from build123d import *

# Parameters (mm, degrees)
SKETCH1_R           = 12.5
SKETCH1_R_2         = 6
SKETCH1_R_3         = 1.5
SKETCH1_R_4         = 3
BOSS_EXTRUDE1_DEPTH = 4.5
BOSS_EXTRUDE2_START = 4.5
SKETCH1_3_R         = 6
SKETCH1_3_R_2       = 3
BOSS_EXTRUDE2_DEPTH = 4.5


with BuildPart() as part:
    # Sketch1 → Boss-Extrude1 (new body)
    # profile 1 of 2: a face of its own
    with BuildSketch(Plane(origin=(0, 0, 0), x_dir=(1, 0, 0), z_dir=(0, 1, 0))):
        with Locations(Location((0, 0, 0), (0, 0, 270))):
            Circle(SKETCH1_R)
        Circle(SKETCH1_R_2, mode=Mode.SUBTRACT)
        with Locations(Location((-8.227241336, 4.75, 0), (0, 0, 270))):
            Circle(SKETCH1_R_3, mode=Mode.SUBTRACT)
        with Locations(Location((-8.227241336, -4.75, 0), (0, 0, 270))):
            Circle(SKETCH1_R_3, mode=Mode.SUBTRACT)
        with Locations(Location((0, -9.5, 0), (0, 0, 270))):
            Circle(SKETCH1_R_3, mode=Mode.SUBTRACT)
        with Locations(Location((8.227241336, -4.75, 0), (0, 0, 270))):
            Circle(SKETCH1_R_3, mode=Mode.SUBTRACT)
        with Locations(Location((8.227241336, 4.75, 0), (0, 0, 270))):
            Circle(SKETCH1_R_3, mode=Mode.SUBTRACT)
        with Locations(Location((0, 9.5, 0), (0, 0, 270))):
            Circle(SKETCH1_R_3, mode=Mode.SUBTRACT)
    # profile 2 of 2: a face of its own
    with BuildSketch(Plane(origin=(0, 0, 0), x_dir=(1, 0, 0), z_dir=(0, 1, 0))):
        Circle(SKETCH1_R_2)
        with Locations(Location((0, 0, 0), (0, 0, 270))):
            Circle(SKETCH1_R_4, mode=Mode.SUBTRACT)
    extrude(amount=BOSS_EXTRUDE1_DEPTH)

    # Sketch1<3> → Boss-Extrude2 (add)
    with BuildSketch(Plane(origin=(0, 0, 0), x_dir=(1, 0, 0), z_dir=(0, 1, 0)).offset(BOSS_EXTRUDE2_START)):
        with Locations(Location((0, 0, 0), (0, 0, 270))):
            Circle(SKETCH1_3_R)
        with Locations(Location((0, 0, 0), (0, 0, 270))):
            Circle(SKETCH1_3_R_2, mode=Mode.SUBTRACT)
    extrude(amount=BOSS_EXTRUDE2_DEPTH)


solid = part.part
Can you work these out from the model? Positions are in its coordinate system, mm. A direction names the side the tool comes from. Round coordinates to 2 decimals unless told otherwise and drop trailing zeros. Loops run counter-clockwise (first coordinate to the right, second up) from the corner with the lowest first, then second, coordinate; pieces in that order, holes last. Notation, with made-up numbers: (46.5, 68.5) - (50.5, 68.5) arc R32 ccw to (50.5, 97.5) - close; hole circle Ø1 at (36, 80). An arc over 180 degrees is marked (long way). Use CSV: the item, a comma, the result in double quotes. Start each with the question number.
1) If we section it at A-A on z = 0: Write out the boundary of the cut face in (x, y).
2) If we section it at B-B on x = -7.5: Write out the boundary of the cut face in (y, z), plus the area to 3 significant figures.
3) For pin 1 Ø5 at (x, z) = (-4, -8) entering from +Y, with a flat end and sliding along its axis, tell me the tip position at first contact or that it passes through.
4) If we section it at C-C on z = -4.75: Write out the boundary of the cut face in (x, y).
5) We'd pull the mould along X, two halves only. Please class faces 3 (the cylindrical face through (-7.213, 2.218, -5.856)), 4 (the cylindrical face through (3.755, 2.218, 11.923)), 5 (the flat face through (3, 9, 1)), 6 (the cylindrical face through (0.9, 4.44, 2.86)): released by +X, released by -X, zero draft, split by the parting line, or undercut.
6) For faces 1 (the flat face through (5.4, 4.5, -3)), 2 (the cylindrical face through (0, 2, -11)), which set-ups out of +Z, -Z, +X, -X, +Y, -Y let a thin tool reach every point of the face, with its end or its side?
7) Please list where these lines run through material, in increasing order: probe 1 along X at (y, z) = (1.85, 4.75); probe 2 along Z at (x, y) = (8, 2.5); probe 3 along X at (y, z) = (6.25, 0). Write a range as [from, to].
8) If we section it at D-D on x = 2.25: Write out the boundary of the cut face in (y, z).
Geometry results:
1,outline,"(-12.5, 0) - (-3, 0) - (-3, 9) - (-6, 9) - (-6, 4.5) - (-12.5, 4.5) - close; (3, 0) - (12.5, 0) - (12.5, 4.5) - (6, 4.5) - (6, 9) - (3, 9) - close"
2,outline,"(0, -10) - (4.5, -10) - (4.5, -6.06) - (0, -6.06) - close; (0, -3.44) - (4.5, -3.44) - (4.5, 3.44) - (0, 3.44) - close; (0, 6.06) - (4.5, 6.06) - (4.5, 10) - (0, 10) - close"
2,area,"66.4 mm2"
3,pin 1,"stops at y = 4.5"
4,outline,"(-11.56, 0) - (-9.73, 0) - (-9.73, 4.5) - (-11.56, 4.5) - close; (-6.73, 0) - (6.73, 0) - (6.73, 4.5) - (3.67, 4.5) - (3.67, 9) - (-3.67, 9) - (-3.67, 4.5) - (-6.73, 4.5) - close; (9.73, 0) - (11.56, 0) - (11.56, 4.5) - (9.73, 4.5) - close"
5,face 3,"undercut"
5,face 4,"split by the parting line"
5,face 5,"zero draft"
5,face 6,"undercut"
6,face 1,"+Y"
6,face 2,"+Y, -Y"
7,probe 1,"x = [-11.56, -9.73], [-6.73, 6.73], [9.73, 11.56]"
7,probe 2,"z = [-9.6, -6.23], [-3.27, 3.27], [6.23, 9.6]"
7,probe 3,"x = [-6, -3], [3, 6]"
8,outline,"(0, -12.3) - (4.5, -12.3) - (4.5, -5.56) - (9, -5.56) - (9, -1.98) - (0, -1.98) - close; (0, 1.98) - (9, 1.98) - (9, 5.56) - (4.5, 5.56) - (4.5, 12.3) - (0, 12.3) - close"
